Source: CAD feature listing. Evaluate the final solid. Frame: model axes, mm. A direction names the side the tool comes from. Give positions to 0.01 mm unless a question says otherwise; leave off trailing zeros. Loops run counter-clockwise (first coordinate to the right, second up) from the corner with the lowest first, then second, coordinate; pieces in that order, holes last.
```python
from build123d import *
from build123d.topology import SkipClean

# Parameters (mm, degrees)
SKETCH_1_R               = 4
EXTRUDE_1_DEPTH          = 25
CUT_EXTRUDE_1_DEPTH      = 38.512497308
CUT_EXTRUDE_1_DEPTH_BACK = 38.512497308
CUT_EXTRUDE_2_DEPTH      = 38.512497308
CUT_EXTRUDE_2_DEPTH_BACK = 38.512497308


with BuildPart() as part:
    # Sketch 1 → Extrude 1 (new, symmetric)
    with BuildSketch(Plane.XY):
        Circle(SKETCH_1_R)
    extrude(amount=EXTRUDE_1_DEPTH, both=True)

    # Sketch 2 → Revolve 2 (revolve)
    with SkipClean():  # the faces are left unmerged after this step: merging them gives an invalid solid
        with BuildSketch(Plane(origin=(0, 0, 0), x_dir=(1, 0, 0), z_dir=(0, 1, 0))):
            with BuildLine():
                ThreePointArc((6.403124237, 30), (4.527692569, 34.527692569), (0, 36.403124237))
                Line((0, 36.403124237), (0, 33.5))
                ThreePointArc((0, 33.5), (2.474873734, 32.474873734), (3.5, 30))
                ThreePointArc((3.5, 30), (2.474873734, 27.525126266), (0, 26.5))
                Line((0, 26.5), (0, 23.596875763))
                ThreePointArc((0, 23.596875763), (4.527692569, 25.472307431), (6.403124237, 30))
            make_face()
            with BuildLine():
                Line((0, 33.5), (0, 36.403124237))
                ThreePointArc((0, 36.403124237), (-6.403124237, 30), (0, 23.596875763))
                Line((0, 23.596875763), (0, 26.5))
                ThreePointArc((0, 26.5), (-3.5, 30), (0, 33.5))
            make_face()
            with BuildLine():
                ThreePointArc((0, -23.596875763), (-6.403124237, -30), (0, -36.403124237))
                Line((0, -36.403124237), (0, -33.5))
                ThreePointArc((0, -33.5), (-3.5, -30), (0, -26.5))
                Line((0, -26.5), (0, -23.596875763))
            make_face()
            with BuildLine():
                Line((0, -33.5), (0, -36.403124237))
                ThreePointArc((0, -36.403124237), (4.527692569, -34.527692569), (6.403124237, -30))
                ThreePointArc((6.403124237, -30), (4.527692569, -25.472307431), (0, -23.596875763))
                Line((0, -23.596875763), (0, -26.5))
                ThreePointArc((0, -26.5), (2.474873734, -27.525126266), (3.5, -30))
                ThreePointArc((3.5, -30), (2.474873734, -32.474873734), (0, -33.5))
            make_face()
        revolve(axis=Axis((0, 0, -36.403124237), (0, 0, 1)))

    # Sketch 3 → Cut-Extrude 1 (cut, two sides: drawn at the far end of the back side and taken through both)
    with SkipClean():  # the faces are left unmerged after this step: merging them gives an invalid solid
        with BuildSketch(Plane(origin=(0, 0, 0), x_dir=(0, 0, -1), z_dir=(1, 0, 0)).offset(-CUT_EXTRUDE_1_DEPTH_BACK)):
            Polygon((-18, 4), (-25, 1.5), (-38, 1.5), (-38, 8), (-18, 8), align=None)
            Polygon((-18, -8), (-18, -4), (-25, -1.5), (-38, -1.5), (-38, -8), align=None)
        extrude(amount=CUT_EXTRUDE_1_DEPTH + CUT_EXTRUDE_1_DEPTH_BACK, mode=Mode.SUBTRACT)

    # Sketch 4 → Cut-Extrude 2 (cut, two sides: drawn at the far end of the back side and taken through both)
    with SkipClean():  # the faces are left unmerged after this step: merging them gives an invalid solid
        with BuildSketch(Plane(origin=(0, 0, 0), x_dir=(1, 0, 0), z_dir=(0, 1, 0)).offset(-CUT_EXTRUDE_2_DEPTH_BACK)):
            Polygon((4, 18), (1.5, 25), (1.5, 39), (8, 39), (8, 18), align=None)
            Polygon((-8, 18), (-4, 18), (-1.5, 25), (-1.5, 39), (-8, 39), align=None)
        extrude(amount=CUT_EXTRUDE_2_DEPTH + CUT_EXTRUDE_2_DEPTH_BACK, mode=Mode.SUBTRACT)


solid = part.part
```
(1) Section A-A, the plane z = -5. Return the cut outline in (x, y), then the cut area to 3 significant figures.
A:
outline: circle Ø8 at (0, 0)
area: 50.3 mm2
(2) First-contact query: pin 1 (4 mm diameter, centred on y = -4.5, z = 1.5, fed in from +X); pin 2 (3.5 mm diameter, centred on y = -2.5, z = -32.5, fed in from -X); pin 3 (4 mm diameter, centred on x = 0, z = -26.5, fed in from -Y). Flat tips, straight axial feed; report the tip coordinate or a pass-through.
A:
pin 1: stops at x = 3.12
pin 2: stops at x = -1.5
pin 3: stops at y = -6.22
(3) Reachability of faces 1 (the flat face through (-1.5, -1.5, -33)), 2 (the flat face through (1.5, -1.5, -33)), 3 (the cylindrical face through (3.695, -1.532, 0.35)), 4 (the flat face through (-1.5, 1.5, 33)) from +Z, -Z, +X, -X, +Y, -Y: full face, straight path, thin tool, end or side. Return the list, or none.
A:
face 1: -Z, -X, +Y, -Y
face 2: -Z, +X, +Y, -Y
face 3: none
face 4: +Z, +X, -X, +Y
(4) Ray query, line 1 along X through (y, z) = (-0.25, 5); line 2 along Y through (x, z) = (-1.5, 9.5). Return the intervals inside material, ascending.
A:
line 1: x = -3.99 to 3.99
line 2: y = -3.71 to 3.71
